Geometry check sheet. Reference: the model listing, model coordinates, mm. A direction names the side the tool comes from. Round coordinates to 2 decimals unless told otherwise and drop trailing zeros. Loops run counter-clockwise (first coordinate to the right, second up) from the corner with the lowest first, then second, coordinate; pieces in that order, holes last. Notation, with made-up numbers: (69, -8) -> (78, -8) arc R14 ccw to (78, 16) -> close; hole circle Ø11 at (1, 78). An arc over 180 degrees is marked (long way). Use a Markdown table: item, result. Add a question column.
Q1. Set-up check for faces 4 (the face through (-1.38, -6.2, -23.71)), 5 (the face through (-2.461, -4.732, -37.042)): record each of +Z, -Z, +X, -X, +Y, -Y from which the full face is reachable in a straight line by a thin tool's end or side.
Q2. Sectioned sample at C-C, the plane z = -39. Enter the section's corners in (x, y) (1 decimal).
Q3. Material ranges on L1, parallel to Y at x = 0, z = -27.5; L2, parallel to Z at x = 1.25, y = 5.25; L3, parallel to X at y = -2.25, z = -45, recorded low to high.
Q4. Release check for a two-part mould opening along X. For faces 1 (the face through (-3.78, -2.9, -23.42)), 2 (the face through (-4, 3, 0)), 3 (the face through (2.461, -4.732, -10.456)) record: released by +X, released by -X, zero draft, split by the parting line, or undercut.
Q5. Gauge pin test, flat ends, axial feed: P1, Ø3, axis at y = -3, z = -22.5, coming from the -X side; P2, Ø1, axis at y = 3, z = -24.5, coming from the +X side; P3, Ø1.5, axis at x = 4.5, z = -14, coming from the +Y side; P4, Ø5.5, axis at x = 0, y = 0, coming from the -Z side. Record the tip position at first contact, or that the pin passes through.
Q6. Sectioned sample at A-A, the plane x = 0. Enter the section's corners in (y, z), then the cut area to 3 significant figures.
Autodesk Inventor part; units mm, degrees
ref_plane "YZ Plane" through (0, 0, 0) normal (1, 0, 0) x (0, 1, 0)
ref_plane "XZ Plane" through (0, 0, 0) normal (0, 1, 0) x (-1, 0, 0)
ref_plane "XY Plane" through (0, 0, 0) normal (0, 0, 1) x (1, 0, 0)
sketch "Sketch1" plane through (0, 0, 0) normal (0, 0, 1) x (1, 0, 0)
  circle A0 centre (0, 0) radius 6.35
  dimension "d0" = 12.7
extrude "Extrusion1" add sketch "Sketch1" against normal blind 47.498
sketch "Sketch2" plane through (0, 0, 0) normal (0, 0, 1) x (1, 0, 0)
  circle A0 centre (0, 0) radius 6.35
  circle A1 centre (0, 0) radius 5.334
  dimension "d4" = 10.668
extrude "Extrusion2" cut sketch "Sketch2" against normal blind 21.209
sketch "Sketch3" plane through (0, 0, -47.498) normal (0, 0, -1) x (-1, 0, 0)
  circle A0 centre (0, 0) radius 6.35
  circle A1 centre (0, 0) radius 5.334
  dimension "d7" = 10.668
extrude "Extrusion3" cut sketch "Sketch3" against normal blind 21.209
sketch "Sketch4" plane through (0, 0, 0) normal (0, 0, 1) x (1, 0, 0)
  circle A0 centre (0, 0) radius 5.334
  circle A1 centre (0, 0) radius 4.7625
  dimension "d10" = 9.525
extrude "Extrusion4" cut sketch "Sketch4" against normal through all contours A1
properties part number "Cane Adapter"
Values:
| question | item | result |
|---|---|---|
| 1 | face 4 | +Z, -Z |
| 1 | face 5 | -Z |
| 2 | outline | circle Ø10.7 at (0, 0); hole circle Ø9.5 at (0, 0) |
| 3 | L1 | -5.33 to -4.76, 4.76 to 5.33 |
| 3 | L2 | -26.29 to -21.21 |
| 3 | L3 | -4.84 to -4.2, 4.2 to 4.84 |
| 4 | face 1 | undercut |
| 4 | face 2 | zero draft |
| 4 | face 3 | split by the parting line |
| 5 | P1 | x = -6.17 |
| 5 | P2 | x = 5.84 |
| 5 | P3 | y = 3.79 |
| 5 | P4 | through |
| 6 | outline | (-6.35, -26.29) -> (-5.33, -26.29) -> (-5.33, -47.5) -> (-4.76, -47.5) -> (-4.76, 0) -> (-5.33, 0) -> (-5.33, -21.21) -> (-6.35, -21.21) -> close; (4.76, -47.5) -> (5.33, -47.5) -> (5.33, -26.29) -> (6.35, -26.29) -> (6.35, -21.21) -> (5.33, -21.21) -> (5.33, 0) -> (4.76, 0) -> close |
| 6 | area | 64.6 mm^2 |
